```python
from build123d import *

# Parameters (mm, degrees)
SKETCH001_R          = 14
SKETCH002_R          = 14
POCKET_DEPTH         = 14.001
POCKET_DEPTH_BACK    = -14.001
SKETCH003_R          = 1.75
POCKET001_DEPTH      = 15
POCKET001_DEPTH_BACK = -5
POCKET002_DEPTH      = 10
SKETCH005_R          = 5.5
POCKET003_DEPTH      = 3
FILLET_R             = 13


with BuildPart() as part:
    # Sketch → AdditiveLoft section 0
    with BuildSketch(Plane.XY):
        with BuildLine():
            ThreePointArc((14, 0), (0, 14), (-14, 0))
            Line((-14, 0), (-14, -20))
            ThreePointArc((-14, -20), (0, -34), (14, -20))
            Line((14, 0), (14, -20))
        make_face()
    # Sketch001 (on DatumPlane) → AdditiveLoft section 1
    with BuildSketch(Plane.XY.offset(180)):
        Circle(SKETCH001_R)
    loft()

    # Sketch002 (on DatumPlane) → Pocket (cut, two sides)
    with BuildSketch(Plane.YZ) as pocket_sk:
        with Locations((14, 140)):
            Circle(SKETCH002_R)
    extrude(amount=-POCKET_DEPTH, mode=Mode.SUBTRACT)
    extrude(pocket_sk.sketch, amount=-POCKET_DEPTH_BACK, mode=Mode.SUBTRACT)

    # Sketch003 (on DatumPlane) → Pocket001 (cut, two sides)
    with BuildSketch(Plane(origin=(0, 0, 0), x_dir=(-1, 0, 0), z_dir=(0, 1, 0))) as pocket001_sk:
        with Locations((0, 140)):
            Circle(SKETCH003_R)
    extrude(amount=-POCKET001_DEPTH, mode=Mode.SUBTRACT)
    extrude(pocket001_sk.sketch, amount=-POCKET001_DEPTH_BACK, mode=Mode.SUBTRACT)

    # Sketch004 (on DatumPlane) → Pocket002 (cut)
    with BuildSketch(Plane(origin=(0, 0, 3), x_dir=(1, 0, 0), z_dir=(0, 0, -1))):
        with BuildLine():
            ThreePointArc((-5.5, 0), (0, -5.5), (5.5, 0))
            Line((5.5, 0), (5.5, 10))
            ThreePointArc((5.5, 10), (0, 15.5), (-5.5, 10))
            Line((-5.5, 0), (-5.5, 10))
        make_face()
    extrude(amount=-POCKET002_DEPTH, mode=Mode.SUBTRACT)

    # Sketch005 (on Face1 of Pocket002) → Pocket003 (cut)
    with BuildSketch(Plane(origin=(0, 0, 0), x_dir=(1, 0, 0), z_dir=(0, 0, -1))):
        with Locations((0, 10)):
            Circle(SKETCH005_R)
        with BuildLine():
            ThreePointArc((-2, 0), (0, -2), (2, 0))
            Line((2, 0), (2, 10))
            ThreePointArc((2, 10), (0, 12), (-2, 10))
            Line((-2, 0), (-2, 10))
        make_face()
    extrude(amount=-POCKET003_DEPTH, mode=Mode.SUBTRACT)

    # Fillet
    fillet_edges = [part.edges().sort_by_distance(p)[0] for p in [
        (0, 14, 180),
        (-14, 0, 180),
        (0, -14, 180),
        (13.332137, -4.272484, 180),
        (13.332137, 4.272484, 180),
    ]]
    fillet(fillet_edges, radius=FILLET_R)


solid = part.part
```
Here's how the part is built. I have some questions about the finished solid (model axes, mm). A direction names the side the tool comes from. Coordinates: 2 decimals unless noted, no trailing zeros. Return JSON: item names as keys, results as strings.
1) Will these pins go through, and if not, where does the flat tip stop? pin 1 (5.5 mm diameter, centred on x = -2, y = -8.5, fed in from -Z); pin 2 (4 mm diameter, centred on x = 8.5, z = 74.5, fed in from +Y); pin 3 (9 mm diameter, centred on x = 0, y = -10, fed in from +Z); pin 4 (1 mm diameter, centred on x = -3, y = 2.5, fed in from -Z).
Results below:
{"pin 1": "z = 13", "pin 2": "y = 12.3", "pin 3": "z = 179.62", "pin 4": "z = 0"}
2) Thinking about a two-plate mould opening in X: for faces 1 (the face through (3, -15, 0)), 2 (the face through (0, 2, 1)), which applies, +X half, -X half, draft (parallel to the pull), parting line (faces both ways), or undercut?
Results below:
{"face 1": "draft", "face 2": "undercut"}
3) I need wall thicknesses on line 1 (X direction, y = -10, z = 5.75); line 2 (Z direction, x = 2.75, y = -4); line 3 (X direction, y = -5.5, z = 74). Which ranges of each line are inside material? Lowest first, please. Write a range as from..to.
Results below:
{"line 1": "-14..-5.5, 5.5..14", "line 2": "0..3, 13..179.69", "line 3": "-14..14"}
4) For faces 3 (the face through (-2, -2, 1)), 4 (the face through (5.5, -5, 8)), 5 (the face through (0, -15, 140)), which set-ups out of +Z, -Z, +X, -X, +Y, -Y let a thin tool reach every point of the face, with its end or its side?
Results below:
{"face 3": "-Z", "face 4": "none", "face 5": "+Y"}
